Can you work these out from the drawing? Everything is in mm from the part's minimum corner. A direction names the side the tool comes from. Round coordinates to 2 decimals unless told otherwise and drop trailing zeros. Write each loop counter-clockwise with the first axis right and the second up, starting at its lowest first coordinate (ties: lowest second). Pieces come first, ordered by that corner, then holes. Notation, with made-up numbers: (7.5, 39.5) -> (20.5, 39.5) arc R13 ccw to (20.5, 62.5) -> close; hole circle Ø10 at (-12, -25). An arc over 180 degrees is marked (long way). Answer as CSV lines item,"result". Start each with the question number.
Q1. If I drill on line 1 (X direction, y = 2.25, z = 1.5); line 2 (X direction, y = 12.5, z = 3.75) (1 decimal); line 3 (Y direction, x = 9.75, z = 3.5) (1 decimal), over which ranges is the centre line in solid material (lowest first)? Write a range as [from, to].
Q2. Imagine slicing it at D-D on x = 4.25. Please give me the cut outline in (y, z).
Q3. Will these pins go through, and if not, where does the flat tip stop? pin 1 Ø3 at (x, y) = (5.5, 11.5) entering from +Z; pin 2 Ø1.1 at (x, z) = (5.5, 5) entering from -Y; pin 3 Ø3 at (x, z) = (2.5, 1.5) entering from +Y; pin 4 Ø3 at (x, z) = (2, 2) entering from +Y (1 decimal).
Q4. If we mould it in two halves opening along X, with no side actions, what happens to the marked faces 1, 2 and 3? For each: pulls with the +X half, pulls with the -X half, needs draft (parallel to the pull), parting line crosses it, or undercut.
Q5. Imagine slicing it at C-C on z = 8.5. Please give me the cut outline in (x, y).
Q6. Imagine slicing it at B-B on x = 8.25. Please give me the cut outline in (y, z) (1 decimal).
Q7. Imagine slicing it at A-A on y = 2.75. Please give me the cut outline in (x, z).
Q8. For the marked faces 4 and 5, which set-ups out of +Z, -Z, +X, -X, +Y, -Y let a thin tool reach every point of the face, with its end or its side?
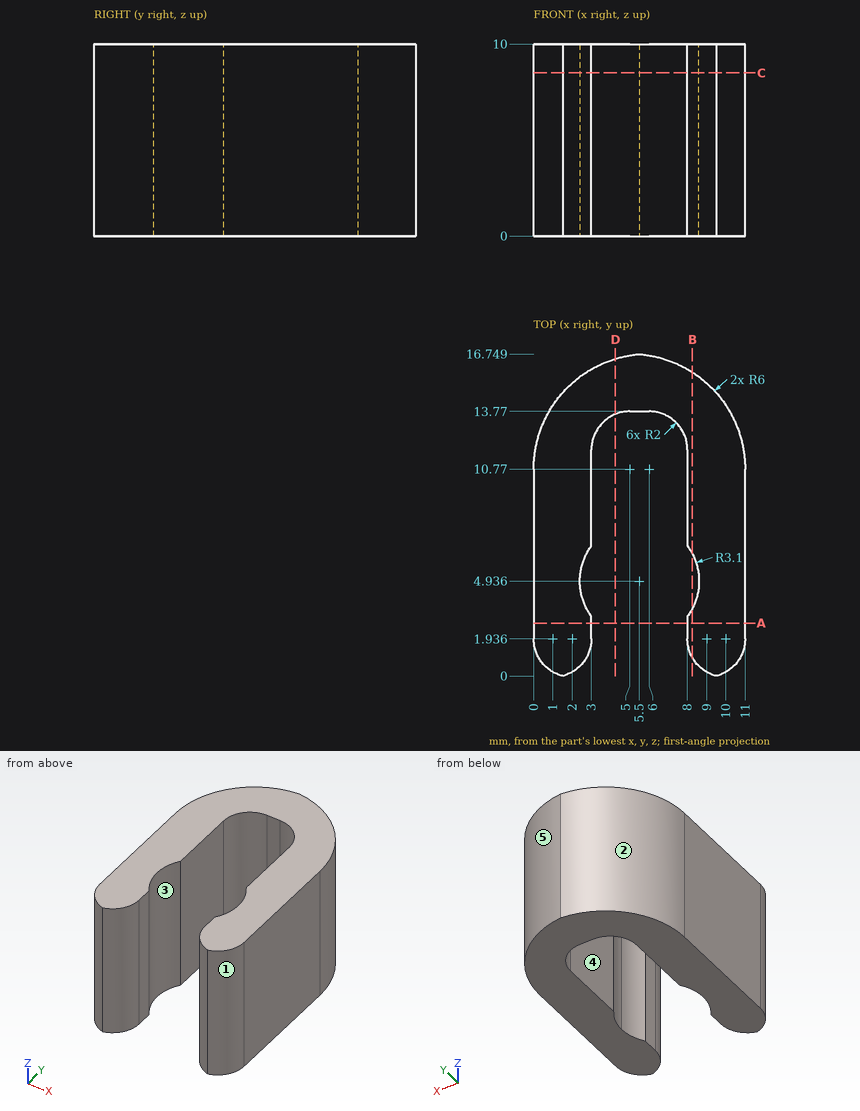
Checks:
1,line 1,"[0, 3], [8, 11]"
1,line 2,"[0.3, 3.1], [7.9, 10.7]"
1,line 3,"[0.1, 14.4]"
2,outline,"(13.62, 0) -> (16.51, 0) -> (16.51, 10) -> (13.62, 10) -> close"
3,pin 1,"through"
3,pin 2,"y = 13.77"
3,pin 3,"y = 16.43"
3,pin 4,"y = 16.2"
4,face 1,"pulls with the +X half"
4,face 2,"pulls with the -X half"
4,face 3,"undercut"
5,outline,"(0, 1.94) arc R2 ccw to (1.5, 0) arc R2 ccw to (3, 1.94) -> (3, 3.1) arc R3.1 cw to (3, 6.77) -> (3, 11.77) arc R2 cw to (5, 13.77) -> (6, 13.77) arc R2 cw to (8, 11.77) -> (8, 6.77) arc R3.1 cw to (8, 3.1) -> (8, 1.94) arc R2 ccw to (9.5, 0) arc R2 ccw to (11, 1.94) -> (11, 10.77) arc R6 ccw to (5.5, 16.75) arc R6 ccw to (0, 10.77) -> close"
6,outline,"(1, 0) -> (3.5, 0) -> (3.5, 10) -> (1, 10) -> close; (6.4, 0) -> (15.8, 0) -> (15.8, 10) -> (6.4, 10) -> close"
7,outline,"(0, 0) -> (3, 0) -> (3, 10) -> (0, 10) -> close; (8, 0) -> (11, 0) -> (11, 10) -> (8, 10) -> close"
8,face 4,"+Z, -Z, -Y"
8,face 5,"+Z, -Z, +X, +Y"
